Autodesk Inventor part; units mm, degrees
ref_plane "YZ Plane" through (0, 0, 0) normal (1, 0, 0) x (0, 1, 0)
ref_plane "XZ Plane" through (0, 0, 0) normal (0, 1, 0) x (-1, 0, 0)
sketch "Sketch1" plane through (0, 0, 0) normal (0, 1, 0) x (-1, 0, 0)
  circle A0 centre (0, 0) radius 17.5
  circle A1 centre (0, 0) radius 5.25
  dimension "d0" = 35
  dimension "d3" = 10.5
extrude "Extrusion1" add sketch "Sketch1" along normal blind 28.3
ref_plane "Work Plane1" through (0, 0, -17.5) normal (0, 0, 1) x (1, 0, 0)
sketch "Sketch2" plane through (0, 0, -17.5) normal (0, 0, 1) x (1, 0, 0)
  line L0 (0, 0) -> (0, 12.5)
  circle A0 centre (0, 12.5) radius 2.25
  dimension "d4" = 12.5
  dimension "d5" = 4.5
extrude "Extrusion2" cut sketch "Sketch2" along normal through all
sketch "Sketch3" plane through (0, 28.3, 0) normal (0, 1, 0) x (1, 0, 0)
  circle A0 centre (0, 0) radius 17.5
extrude "Extrusion3" add sketch "Sketch3" along normal blind 2
sketch "Sketch4" plane through (0, 30.3, 0) normal (0, 1, 0) x (1, 0, 0)
  circle A0 centre (0, 0) radius 2.75
  circle A1 centre (0, 0) radius 7.2188
  dimension "d10" = 5.5
extrude "Extrusion4" add sketch "Sketch4" along normal blind 6 contours A0 | A1
properties part number "StuurPotentiometerConnector"
Input: part model. Units: mm. Frame: model coordinates. A direction names the side the tool comes from. Round coordinates to 2 decimals unless told otherwise and drop trailing zeros. Write each loop counter-clockwise with the first axis right and the second up, starting at its lowest first coordinate (ties: lowest second). Pieces come first, ordered by that corner, then holes. Notation, with made-up numbers: M -10.75,-3 L 22.25,-3 A36 ccw 22.25,32 Z; hole C 51,55.5 d5. An arc over 180 degrees is marked long. Write each question's results on one line, items separated by ' | '.
Q1. Line query: line 1 along Y through (x, z) = (0, -8); line 2 along Y through (x, z) = (-4, -9); line 3 along X through (y, z) = (12.5, 9.75). Output: solid intervals per line, ascending.
Results:
line 1: y = 0 to 10.25, 14.75 to 30.3 | line 2: y = 0 to 30.3 | line 3: x = -14.53 to -2.25, 2.25 to 14.53
Q2. Section query B-B (y = 13). Return loops of the section in (x, z), and give its area (3 significant figures).
Results:
outline: M -2.19,-17.36 L -2.19,-4.77 A5.25 cw -2.19,4.77 L -2.19,17.36 A17.5 ccw Z; M 2.19,-17.36 A17.5 ccw 2.19,17.36 L 2.19,4.77 A5.25 cw 2.19,-4.77 Z | area: 767 mm^2
Q3. Section query D-D (z = 8.5). Return loops of the section in (x, y).
Results:
outline: M -15.3,0 L 15.3,0 L 15.3,30.3 L -15.3,30.3 Z; hole C 0,12.5 d4.5
Q4. Pin query (flat end, axial travel): P1, Ø2, axis at x = 4, y = 10.5, coming from the -Z side; P2, Ø6, axis at y = 18.5, z = -11, coming from the -X side; P3, Ø1, axis at x = -9.5, z = 9, coming from the +Y side; P4, Ø2.5, axis at x = 0, y = 12.5, coming from the +Z side. Return the tip coordinate at first contact, or that it passes through.
Results:
P1: stops at z = -17.24 | P2: stops at x = -15.56 | P3: stops at y = 30.3 | P4: passes through
Q5. Draft query along Y for faces 4 (the face through (-5, 14, -1.6)), 5 (the face through (-0.29, 10.27, 11.03)), 6 (the face through (0, 36.3, 0)). Return one class per face: released by +Y, released by -Y, zero draft, split by the parting line, or undercut.
Results:
face 4: zero draft | face 5: undercut | face 6: released by +Y
Q6. Section query A-A (x = 0). Return loops of the section in (y, z), and give its area (3 significant figures).
Results:
outline: M 0,-17.5 L 10.25,-17.5 L 10.25,-5.25 L 0,-5.25 Z; M 0,5.25 L 10.25,5.25 L 10.25,17.5 L 0,17.5 Z; M 14.75,-17.5 L 30.3,-17.5 L 30.3,-7.22 L 36.3,-7.22 L 36.3,7.22 L 30.3,7.22 L 30.3,17.5 L 14.75,17.5 L 14.75,5.25 L 28.3,5.25 L 28.3,-5.25 L 14.75,-5.25 Z | area: 740 mm^2
Q7. Section query C-C (z = 0). Return loops of the section in (x, y), and give its area (3 significant figures).
Results:
outline: M -17.5,0 L -5.25,0 L -5.25,28.3 L 5.25,28.3 L 5.25,0 L 17.5,0 L 17.5,30.3 L 7.22,30.3 L 7.22,36.3 L -7.22,36.3 L -7.22,30.3 L -17.5,30.3 Z | area: 850 mm^2
Q8. Access query for faces 1 (the face through (4, 0, -4)), 2 (the face through (0, 28.3, 0)), 3 (the face through (6.885, 33.258, 2.168)). Directions: +Z, -Z, +X, -X, +Y, -Y. A direction counts if a zero-diameter tool reaches every point of the face in a straight line with its end or side. Return the directions, or none.
Results:
face 1: +Z, -Z, +X, -X, -Y | face 2: -Y | face 3: +Y
